Input: part model. Units: mm. Frame: model coordinates. Face numbers are marked on the shaded views. A direction names the side the tool comes from. Coordinates: 2 decimals unless noted, no trailing zeros. Order: outer loops, then holes, each group sorted by start corner. A loop starts at its lowest first (then second) coordinate and runs counter-clockwise, first axis right, second up. Notation, with made-up numbers: (10, 1) - (24, 1) arc R23 ccw to (24, 21) - close; hole circle Ø1 at (16, 26). An arc over 180 degrees is marked (long way). One line per question, with ' | ' between items. Start each with the question number.
```python
from build123d import *

# Parameters (mm, degrees)
SKETCH2_R           = 10
BOSS_EXTRUDE1_DEPTH = 24
CUT_EXTRUDE1_REACH  = 32
SKETCH3_R           = 3.5
CUT_EXTRUDE2_REACH  = 32
SKETCH4_R           = 3.5


with BuildPart() as part:
    # Sketch2 → Boss-Extrude1 (new body)
    with BuildSketch(Plane.XY):
        with BuildLine():
            Line((-15, 0), (-15, -15))
            Line((-15, -15), (-15, -42))
            Line((-15, -42), (-11, -42))
            Line((-11, -42), (-11, -10.198039027))
            ThreePointArc((-11, -10.198039027), (0, -15), (11, -10.198039027))
            Line((11, -10.198039027), (11, -42))
            Line((11, -42), (15, -42))
            Line((15, -42), (15, -22))
            Line((15, -22), (15, 0))
            ThreePointArc((15, 0), (0, 15), (-15, 0))
        make_face()
        Circle(SKETCH2_R, mode=Mode.SUBTRACT)
    extrude(amount=BOSS_EXTRUDE1_DEPTH)

    # Sketch3 → Cut-Extrude1 (cut, up to next)
    with BuildSketch(Plane.ZY.offset(15), mode=Mode.PRIVATE) as cut_extrude1_sk1:
        with Locations((12, -33.467780556)):
            Circle(SKETCH3_R)
    cut_extrude1_tool1 = extrude(cut_extrude1_sk1.sketch, amount=-CUT_EXTRUDE1_REACH, mode=Mode.PRIVATE) & part.part
    add(cut_extrude1_tool1.solids().sort_by_distance((-15, -33.467781, 12))[0], mode=Mode.SUBTRACT)
    # Sketch3 → Cut-Extrude1 (cut, up to next)
    with BuildSketch(Plane.ZY.offset(15), mode=Mode.PRIVATE) as cut_extrude1_sk2:
        with BuildLine():
            Line((0, -10.198039027), (4.341204442, -34.818232852))
            ThreePointArc((4.341204442, -34.818232852), (12, -41.244725381), (19.658795558, -34.818232852))
            Line((19.658795558, -34.818232852), (24, -10.198039027))
            Line((24, -10.198039027), (24, -42))
            Line((24, -42), (0, -42))
            Line((0, -42), (0, -10.198039027))
        make_face()
    cut_extrude1_tool2 = extrude(cut_extrude1_sk2.sketch, amount=-CUT_EXTRUDE1_REACH, mode=Mode.PRIVATE) & part.part
    add(cut_extrude1_tool2.solids().sort_by_distance((-15, -22.57732, 1.778238))[0], mode=Mode.SUBTRACT)

    # Sketch4 → Cut-Extrude2 (cut, up to next)
    with BuildSketch(Plane(origin=(15, 0, 0), x_dir=(0, 0, -1), z_dir=(1, 0, 0)), mode=Mode.PRIVATE) as cut_extrude2_sk1:
        with Locations((-12, -33.467780556)):
            Circle(SKETCH4_R)
    cut_extrude2_tool1 = extrude(cut_extrude2_sk1.sketch, amount=-CUT_EXTRUDE2_REACH, mode=Mode.PRIVATE) & part.part
    add(cut_extrude2_tool1.solids().sort_by_distance((15, -33.467781, 12))[0], mode=Mode.SUBTRACT)
    # Sketch4 → Cut-Extrude2 (cut, up to next)
    with BuildSketch(Plane(origin=(15, 0, 0), x_dir=(0, 0, -1), z_dir=(1, 0, 0)), mode=Mode.PRIVATE) as cut_extrude2_sk2:
        with BuildLine():
            Line((0, -10.198039027), (-4.341204442, -34.818232852))
            ThreePointArc((-4.341204442, -34.818232852), (-12, -41.244725381), (-19.658795558, -34.818232852))
            Line((-19.658795558, -34.818232852), (-24, -10.198039027))
            Line((-24, -10.198039027), (-24, -42))
            Line((-24, -42), (0, -42))
            Line((0, -42), (0, -10.198039027))
        make_face()
    cut_extrude2_tool2 = extrude(cut_extrude2_sk2.sketch, amount=-CUT_EXTRUDE2_REACH, mode=Mode.PRIVATE) & part.part
    add(cut_extrude2_tool2.solids().sort_by_distance((15, -22.57732, 1.778238))[0], mode=Mode.SUBTRACT)


solid = part.part
```
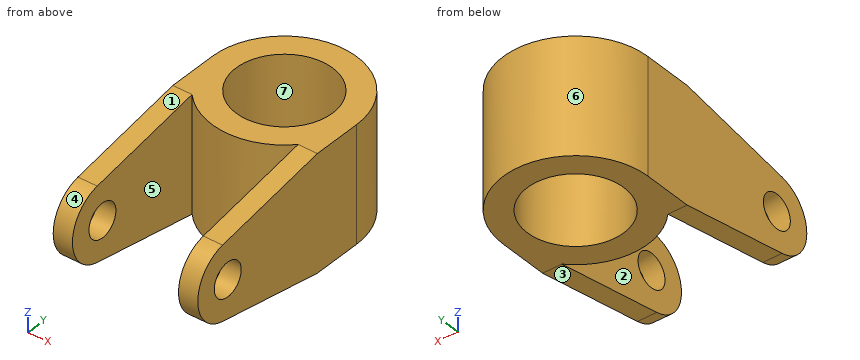
(1) Reachability of the marked faces 1, 2 and 3 from +Z, -Z, +X, -X, +Y, -Y: full face, straight path, thin tool, end or side. Return the list, or none.
(2) Material intervals for line 1 along X through (y, z) = (-23, 18.25); line 2 along Y through (x, z) = (-0.5, 19.25); line 3 along X through (y, z) = (9, 20.75), sorted ascending. Write a range as from..to.
(3) Section D-D (z = 22). Output: boundary loops of the cut face in (x, y).
(4) Draft query along X for the marked faces 4, 5, 6 and 7. Return one class per face: +X half, -X half, draft (parallel to the pull), parting line (faces both ways), or undercut.
(5) Section C-C (x = -12). Output: boundary loops of the cut face in (y, z), then the cut area to 3 significant figures.
(6) Pin query (flat end, axial travel): pin 1 (1 mm diameter, centred on x = -6.5, z = 19.5, fed in from +Y); pin 2 (8 mm diameter, centred on y = -33.47, z = 12, fed in from -X); pin 3 (5 mm diameter, centred on y = 6, z = 21, fed in from -X); pin 4 (3 mm diameter, centred on x = -6, z = 13.5, fed in from +Y). Return the tip coordinate at first contact, or that it passes through.
(7) Section B-B (y = -5.5). Output: boundary loops of the cut face in (x, z), then the cut area to 3 significant figures.
(8) Section A-A (z = 12). Output: boundary loops of the cut face in (x, y).
Worked answers:
1) face 1: +Z, -X, -Y | face 2: +Z, -Z, -Y | face 3: -Z, +X, -Y
2) line 1: x = -15..-11, 11..15 | line 2: y = -14.99..-9.99, 9.99..14.99 | line 3: x = -12..-4.36, 4.36..12
3) outline: (-15, -21.54) - (-11, -21.54) - (-11, -10.2) arc R15 ccw to (11, -10.2) - (11, -21.54) - (15, -21.54) - (15, 0) arc R15 ccw to (-15, 0) - close; hole circle Ø20 at (0, 0)
4) face 4: draft | face 5: undercut | face 6: parting line | face 7: undercut
5) outline: (-34.82, 4.34) - (-10.2, 0) - (9, 0) - (9, 24) - (-10.2, 24) - (-34.82, 19.66) arc R7.78 ccw to start; hole circle Ø7 at (-33.47, 12) | area: 980 mm²
6) pin 1: stops at y = 13.75 | pin 2: stops at x = -15 | pin 3: stops at x = -14.59 | pin 4: stops at y = 14.31
7) outline: (-15, 0) - (-8.35, 0) - (-8.35, 24) - (-15, 24) - close; (8.35, 0) - (15, 0) - (15, 24) - (8.35, 24) - close | area: 319 mm²
8) outline: (-15, -41.24) - (-11, -41.24) - (-11, -36.97) - (-15, -36.97) - close; (-15, -29.97) - (-11, -29.97) - (-11, -10.2) arc R15 ccw to (11, -10.2) - (11, -29.97) - (15, -29.97) - (15, 0) arc R15 ccw to (-15, 0) - close; (11, -41.24) - (15, -41.24) - (15, -36.97) - (11, -36.97) - close; hole circle Ø20 at (0, 0)
